Part model, mm, in its own coordinate system. Coordinates: 2 decimals unless noted, no trailing zeros. Order: outer loops, then holes, each group sorted by start corner. A loop starts at its lowest first (then second) coordinate and runs counter-clockwise, first axis right, second up. Notation, with made-up numbers: M 40,-15.5 L 92,-15.5 A26 cw 92,4.5 Z; hole C -28.75,-16 d6. An arc over 180 degrees is marked long. Write item = value, one per line. Start each with the question number.
from build123d import *

# Parameters (mm, degrees)
F0_W     = 30
F0_H     = 40
F0_R     = 1
F1_DEPTH = 3
F2_R     = 1


# Not quite as in the source:
# - a feature names something its author has since deleted; it is built from what else it names


with BuildPart() as f1:
    # F0 (on Top) → F1 (new body)
    with BuildSketch(Plane.XY):
        Rectangle(F0_W, F0_H)
        with Locations((-9, -12.5)):
            Circle(F0_R, mode=Mode.SUBTRACT)
        with Locations((0, -12.5)):
            Circle(F0_R, mode=Mode.SUBTRACT)
        with Locations((-9, 12.5)):
            Circle(F0_R, mode=Mode.SUBTRACT)
        with Locations((0, 12.5)):
            Circle(F0_R, mode=Mode.SUBTRACT)
    extrude(amount=-F1_DEPTH)

    # F2
    f2_edges = [f1.edges().sort_by_distance(p)[0] for p in [
        (-15, 0, 0),
        (0, 20, 0),
        (15, 0, 0),
        (0, -20, 0),
        (15, 0, -3),
    ]]
    fillet(f2_edges, radius=F2_R)


solid = f1.part
Item 1: Cut at C-C, the plane z = -0.45. Write the cut outline in (x, y), and give its area (3 significant figures).
Item 2: Wall check: line 1 along Y through (x, z) = (0, -1.6); line 2 along Y through (x, z) = (-9.5, -2.55); line 3 along X through (y, z) = (8, -0.45). Give the ranges that are in metal, low to high. Write a range as [from, to].
Item 3: Cut at A-A, the plane x = 0. Write the cut outline in (y, z), and give its area (3 significant figures).
Item 4: Cut at B-B, the plane y = 12.5. Write the cut outline in (x, z).
Item 5: Flat gauge pin, fed straight in: pin 1 (5 mm diameter, centred on x = -0.5, y = -5.5, fed in from +Z). Where does the tip first touch, or does it go through?
Item 6: Pull direction Y, two halves, no side cores. Call faces 1 (the cylindrical face through (0.21, -19.715, -0.301)), 2 (the cylindrical face through (-9.8, 11.9, -1.5)), 3 (the cylindrical face through (0.46, -13.39, -1.48)), 4 (the cylindrical face through (14.715, 0.28, -0.301)): pulls with the +Y half, pulls with the -Y half, needs draft (parallel to the pull), parting line crosses it, or undercut.
Filled sheet:
q1.outline = M -14.84,-19.84 L 14.84,-19.84 L 14.84,19.84 L -14.84,19.84 Z; hole C -9,-12.5 d2; hole C -9,12.5 d2; hole C 0,-12.5 d2; hole C 0,12.5 d2
q1.area = 1,160 mm2
q2.line_1 = [-20, -13.5], [-11.5, 11.5], [13.5, 20]
q2.line_2 = [-20, -13.37], [-11.63, 11.63], [13.37, 20]
q2.line_3 = [-14.84, 14.84]
q3.outline = M -20,-3 L -13.5,-3 L -13.5,0 L -19,0 A1 ccw -20,-1 Z; M -11.5,-3 L 11.5,-3 L 11.5,0 L -11.5,0 Z; M 13.5,-3 L 20,-3 L 20,-1 A1 ccw 19,0 L 13.5,0 Z
q3.area = 108 mm2
q4.outline = M -15,-3 L -10,-3 L -10,0 L -14,0 A1 ccw -15,-1 Z; M -8,-3 L -1,-3 L -1,0 L -8,0 Z; M 1,-3 L 14,-3 A1 ccw 15,-2 L 15,-1 A1 ccw 14,0 L 1,0 Z
q5.pin_1 = 0
q6.face_1 = pulls with the -Y half
q6.face_2 = undercut
q6.face_3 = undercut
q6.face_4 = needs draft
